For this review, use the dimensioned drawing (mm, ordinates from the lowest corner) and the shaded views. A direction names the side the tool comes from. Coordinates: 2 decimals unless noted, no trailing zeros. Order: outer loops, then holes, each group sorted by start corner. A loop starts at its lowest first (then second) coordinate and runs counter-clockwise, first axis right, second up. Notation, with made-up numbers: M -8.5,78 L 14.5,78 A5 cw 14.5,86 Z; hole C 47,60 d9. An arc over 180 degrees is marked long. Answer as CSV lines item,"result". Start each with the question number.
Q1. Consider section C-C on x = 20. Write out the cut boundary in (y, z).
Q2. Wall thickness on L1, parallel to Y at x = 25, z = 64; L2, parallel to X at y = 43, z = 32 (1 decimal); L3, parallel to X at y = 45, z = 40 (1 decimal): over which ranges is each line inside the solid? List them lowest first. Write a range as [from, to].
Q3. Consider section B-B on x = 47.5. Write out the cut boundary in (y, z).
Q4. For P1, Ø18.5, axis at x = 44.68, z = 39.03, coming from the -Y side, flat-tipped, find the tip position at first contact; note if it passes through.
Q5. The part is to be moulded in two halves that separate along Z. For the marked faces 1, 2, 3 and 4, say which applies: +Z half, -Z half, draft (parallel to the pull), parting line (faces both ways), or undercut.
Q6. Machinability: for the marked faces 5 and 6, which of the approach directions +Z, -Z, +X, -X, +Y, -Y give a long, thin tool a straight path to every point of the face, cutting with its end or side? Answer none if there is none.
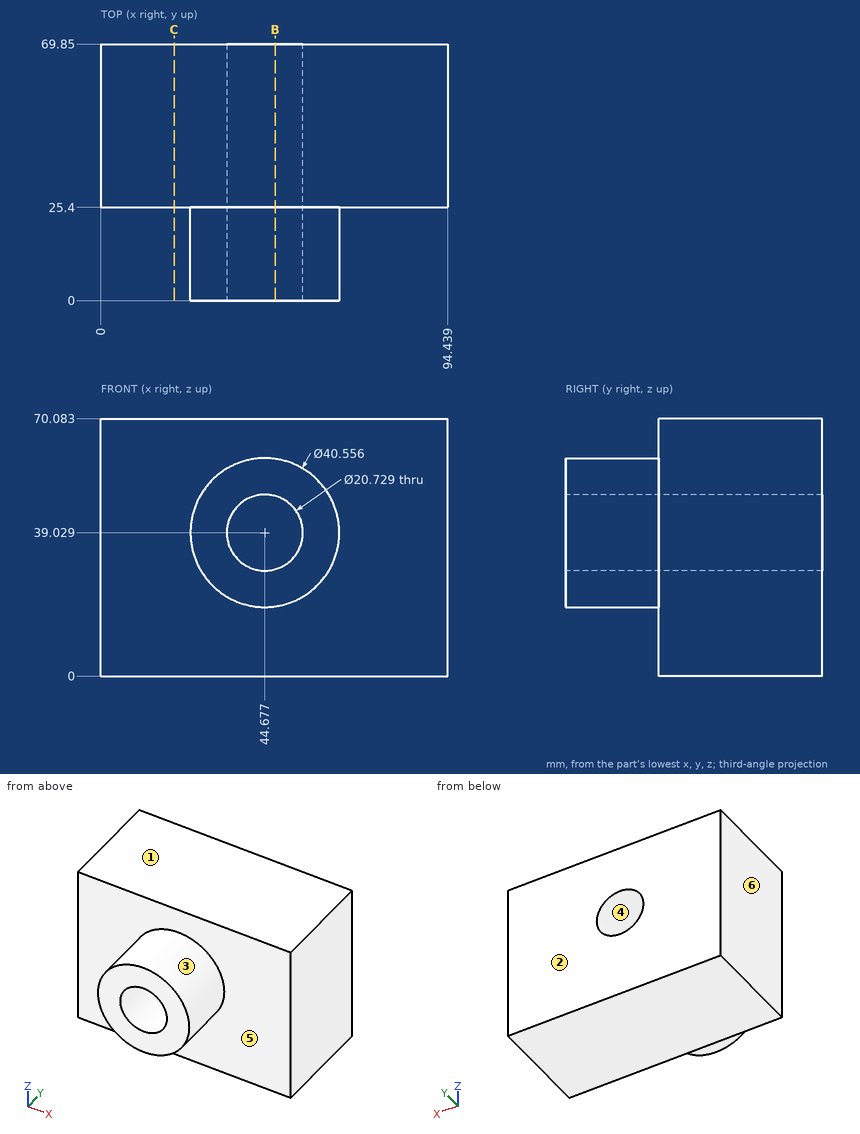
Evaluation:
1,outline,"M 25.4,0 L 69.85,0 L 69.85,70.08 L 25.4,70.08 Z"
2,L1,"y = [25.4, 69.85]"
2,L2,"x = [0, 37.1], [52.3, 94.4]"
2,L3,"x = [0, 34.4], [55, 94.4]"
3,outline,"M 0,18.95 L 25.4,18.95 L 25.4,0 L 69.85,0 L 69.85,29.06 L 0,29.06 Z; M 0,49 L 69.85,49 L 69.85,70.08 L 25.4,70.08 L 25.4,59.11 L 0,59.11 Z"
4,P1,"passes through"
5,face 1,"+Z half"
5,face 2,"draft"
5,face 3,"parting line"
5,face 4,"undercut"
6,face 5,"-Y"
6,face 6,"+Z, -Z, -X, +Y, -Y"
